Can you work these out from the drawing? Everything is in mm from the part's minimum corner. Give positions to 0.01 mm unless a question says otherwise; leave off trailing zeros. Write each loop counter-clockwise with the first axis right and the second up, starting at its lowest first coordinate (ties: lowest second). Pieces come first, ordered by that corner, then holes. Notation, with made-up numbers: (-2, 27.5) - (50, 27.5) arc R24 cw to (50, 62.5) - close; hole circle Ø11 at (51.5, 32). An arc over 180 degrees is marked (long way). Use a Markdown table: item, result. Add a question column.
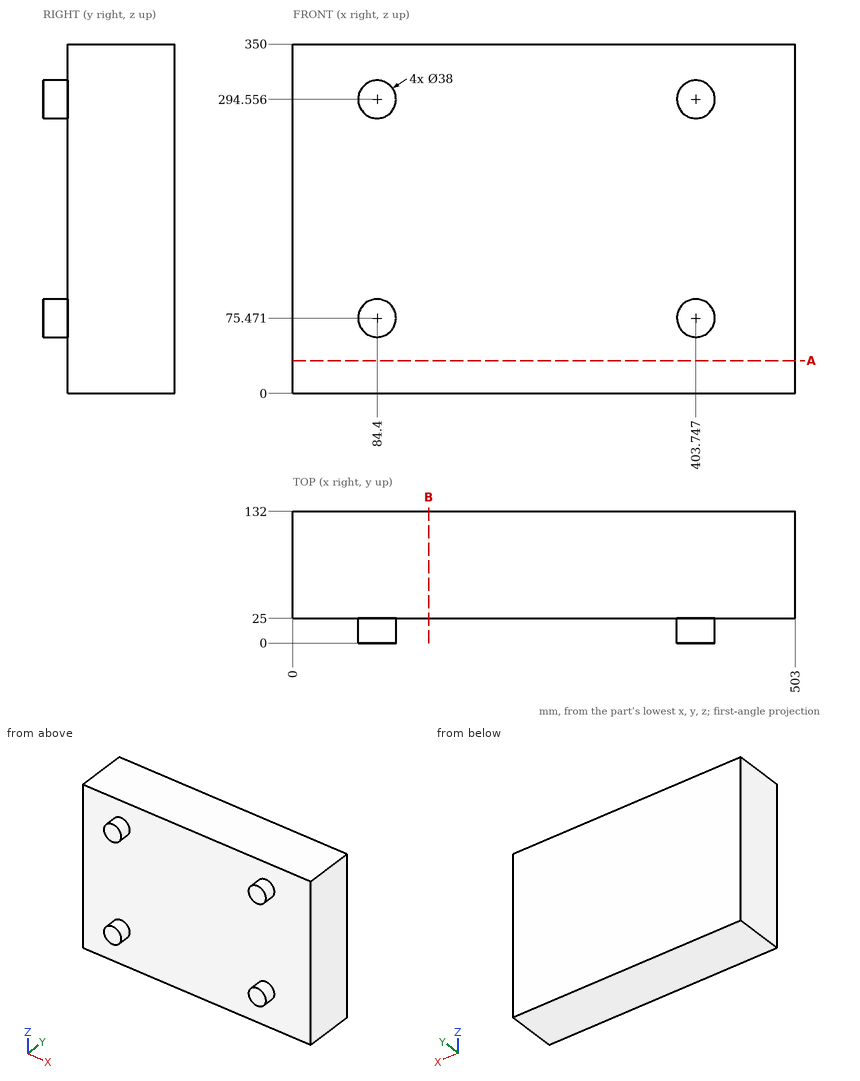
Q1. Suppose I cut it at B-B (x = 136). Please give me the cut outline in (y, z).
Q2. If I drill on probe 1 along Y at (x, z) = (42, 237.5), over which ranges is the centre line in solid material (lowest first)? Write a range as [from, to].
Q3. I'm going to push flat-ended pins straight in: P1, Ø3, axis at x = 306, z = 247.5, coming from the -Y side; P2, Ø10, axis at x = 94.5, y = 15, coming from the -Z side; P3, Ø2, axis at x = 102.5, y = 104, coming from the -Z side. Where does each tip first touch, or does it pass through?
Q4. Suppose I cut it at A-A (z = 33). Please give me the cut outline in (x, y).
Derived:
| question | item | result |
|---|---|---|
| 1 | outline | (25, 0) - (132, 0) - (132, 350) - (25, 350) - close |
| 2 | probe 1 | [25, 132] |
| 3 | P1 | y = 25 |
| 3 | P2 | z = 57.17 |
| 3 | P3 | z = 0 |
| 4 | outline | (0, 25) - (503, 25) - (503, 132) - (0, 132) - close |
